Could you check a few things on this model? Use its own coordinates, in mm. A direction names the side the tool comes from. Round coordinates to 2 decimals unless told otherwise and drop trailing zeros. Loops run counter-clockwise (first coordinate to the right, second up) from the corner with the lowest first, then second, coordinate; pieces in that order, holes last. Notation, with made-up numbers: (-26, 50) - (-2, 50) arc R19 cw to (-2, 66) - close; hole circle Ø3 at (41.25, -17). An arc over 180 degrees is marked (long way). Answer as CSV lines item,"result". Start each with the question number.
1) Suppose I cut it at B-B, the plane z = 140.5. Write out the boundary of the cut face in (x, y), then the cut area to 3 significant figures.
2) Please list where these lines run through material, in increasing order: line 1 along X through (y, z) = (12, 244); line 2 along Y through (x, z) = (0, 342); line 3 along Z through (x, y) = (0, -16.6).
3) Suppose I cut it at A-A, the plane x = 0. Write out the boundary of the cut face in (y, z), then the cut area to 3 significant figures.
4) We'd pull the mould along Z, two halves only. Please class faces 1 (the face through (0, -16, 480)), 2 (the face through (0, 14.4, 243)), 3 (the face through (0, 16, 454)), 4 (the face through (0, -16, 0)): pulls with the +Z half, pulls with the -Z half, needs draft (parallel to the pull), parting line crosses it, or undercut.
5) Which directions (+Z, -Z, +X, -X, +Y, -Y) give clear straight access to the entire face, cutting with the end or side of a thin tool? Please do faces 5 (the face through (20, 0, 232)), 6 (the face through (-16, 0, 217)), 7 (the face through (27, 9, 2)).
6) I'm going to push flat-ended pins straight in: pin 1 Ø3 at (y, z) = (-7.5, 224) entering from +X; pin 2 Ø3 at (x, y) = (18.5, -0.5) entering from +Z; pin 3 Ø15.5 at (x, z) = (0, 460) entering from +Y; pin 4 Ø1.2 at (x, y) = (22, 4) entering from +Z. Where does each tip first touch, or does it pass through?
```python
from build123d import *

# Parameters (mm, degrees)
SKETCH1_W               = 40
SKETCH1_H               = 36
SKETCH1_W_2             = 32
SKETCH1_H_2             = 28.8
BOSS_EXTRUDE1_DEPTH     = 480
SKETCH2_W               = 50
SKETCH2_H               = 28.8
CUT_EXTRUDE1_DEPTH      = 40
FILLET2_RADIUS          = 20
FILLET2_LENGTH          = 3.6
FILLET3_RADIUS          = 20
FILLET3_LENGTH          = 3.6
CUT_EXTRUDE2_DEPTH      = 482.763427421
CUT_EXTRUDE2_DEPTH_BACK = 482.763427421
SKETCH3_R               = 6
SKETCH4_R               = 2.5
BOSS_EXTRUDE2_DEPTH     = 36
CUT_EXTRUDE3_START      = 9
SKETCH5_R               = 5
CUT_EXTRUDE3_DEPTH      = 9
CUT_EXTRUDE4_START      = -9
SKETCH7_R               = 5
CUT_EXTRUDE4_DEPTH      = 9


with BuildPart() as part:
    # Sketch1 → Boss-Extrude1 (new body)
    with BuildSketch(Plane.XY):
        Rectangle(SKETCH1_W, SKETCH1_H)
        Rectangle(SKETCH1_W_2, SKETCH1_H_2, mode=Mode.SUBTRACT)
    extrude(amount=BOSS_EXTRUDE1_DEPTH)

    # Sketch2 → Cut-Extrude1 (cut)
    with BuildSketch(Plane.XY.offset(480)):
        Rectangle(SKETCH2_W, SKETCH2_H)
    extrude(amount=-CUT_EXTRUDE1_DEPTH, mode=Mode.SUBTRACT)

    # Fillet2: full round fillet: the end face becomes a half cylinder, R = half its width
    fillet2_face = Plane((0, -16.2, 480), x_dir=(0, -1, 0), z_dir=(0, 0, 1))  # on the end face: x along it, z out of the body
    fillet2_slab = fillet2_face.offset(-FILLET2_RADIUS / 2) * Box(FILLET2_LENGTH, 2 * FILLET2_RADIUS, FILLET2_RADIUS, mode=Mode.PRIVATE)  # the body's end, R deep
    fillet2_round = Plane((0, -16.2, 460), x_dir=(0, 0, 1), z_dir=(0, -1, 0)) * Cylinder(FILLET2_RADIUS, FILLET2_LENGTH, mode=Mode.PRIVATE)  # its axis R under the face
    add(fillet2_slab - fillet2_round, mode=Mode.SUBTRACT)

    # Fillet3: full round fillet: the end face becomes a half cylinder, R = half its width
    fillet3_face = Plane((0, 16.2, 480), x_dir=(0, -1, 0), z_dir=(0, 0, 1))  # on the end face: x along it, z out of the body
    fillet3_slab = fillet3_face.offset(-FILLET3_RADIUS / 2) * Box(FILLET3_LENGTH, 2 * FILLET3_RADIUS, FILLET3_RADIUS, mode=Mode.PRIVATE)  # the body's end, R deep
    fillet3_round = Plane((0, 16.2, 460), x_dir=(0, 0, 1), z_dir=(0, -1, 0)) * Cylinder(FILLET3_RADIUS, FILLET3_LENGTH, mode=Mode.PRIVATE)  # its axis R under the face
    add(fillet3_slab - fillet3_round, mode=Mode.SUBTRACT)

    # Sketch3 → Cut-Extrude2 (cut, two sides: drawn at the far end of the back side and taken through both)
    with BuildSketch(Plane(origin=(0, 18, 0), x_dir=(1, 0, 0), z_dir=(0, 1, 0)).offset(-CUT_EXTRUDE2_DEPTH_BACK)):
        with Locations(Location((0, -460, 0), (0, 0, 270))):
            Circle(SKETCH3_R)
    extrude(amount=CUT_EXTRUDE2_DEPTH + CUT_EXTRUDE2_DEPTH_BACK, mode=Mode.SUBTRACT)

    # Sketch4 → Boss-Extrude2 (add)
    with BuildSketch(Plane.XZ.offset(18)):
        with BuildLine():
            Line((20, 0), (20, 10.898129461))
            Line((20, 10.898129461), (22.5, 10.898129461))
            Line((22.5, 10.898129461), (22.5, 4.330127019))
            ThreePointArc((22.5, 4.330127019), (29.330127019, -2.5), (20, 0))
        make_face()
        with Locations(Location((25, 0, 0), (0, 0, 270))):
            Circle(SKETCH4_R, mode=Mode.SUBTRACT)
    extrude(amount=-BOSS_EXTRUDE2_DEPTH)

    # Sketch5 → Cut-Extrude3 (cut)
    with BuildSketch(Plane(origin=(0, -9, 0), x_dir=(-1, 0, 0), z_dir=(0, -1, 0)).offset(CUT_EXTRUDE3_START)):
        with Locations((-25, 0)):
            Circle(SKETCH5_R)
    extrude(amount=-CUT_EXTRUDE3_DEPTH, mode=Mode.SUBTRACT)

    # Sketch7 → Cut-Extrude4 (cut)
    with BuildSketch(Plane(origin=(0, 9, 0), x_dir=(1, 0, 0), z_dir=(0, 1, 0)).offset(CUT_EXTRUDE4_START)):
        with Locations((25, 0)):
            Circle(SKETCH7_R)
    extrude(amount=CUT_EXTRUDE4_DEPTH, mode=Mode.SUBTRACT)


solid = part.part
```
Filled sheet:
1,outline,"(-20, -18) - (20, -18) - (20, 18) - (-20, 18) - close; hole (-16, -14.4) - (16, -14.4) - (16, 14.4) - (-16, 14.4) - close"
1,area,"518 mm²"
2,line 1,"-20 to -16, 16 to 20"
2,line 2,"-18 to -14.4, 14.4 to 18"
2,line 3,"0 to 454, 466 to 480"
3,outline,"(-18, 0) - (-14.4, 0) - (-14.4, 454) - (-18, 454) - close; (-18, 466) - (-14.4, 466) - (-14.4, 480) - (-18, 480) - close; (14.4, 0) - (18, 0) - (18, 454) - (14.4, 454) - close; (14.4, 466) - (18, 466) - (18, 480) - (14.4, 480) - close"
3,area,"3,370 mm²"
4,face 1,"pulls with the +Z half"
4,face 2,"needs draft"
4,face 3,"undercut"
4,face 4,"pulls with the -Z half"
5,face 5,"+Z, +X, +Y, -Y"
5,face 6,"+Z, -Z"
5,face 7,"-Z, +X"
6,pin 1,"x = 20"
6,pin 2,"z = 440"
6,pin 3,"y = 18"
6,pin 4,"z = 10.9"
